Could you check a few things on this model? Use its own coordinates, in mm. Round coordinates to 2 decimals unless told otherwise and drop trailing zeros. Write each question's results on one line, items separated by ' | '. Start each with the question number.
(1) Imagine slicing it at A-A on z = 7.25. State how many separate pieces and enclosed holes the cut face has, then the cut area to 3 significant figures.
(2) Please list where these lines run through material, in increasing order: line 1 (Y direction, x = 162, z = 3); line 2 (X direction, y = 149.5, z = 6); line 3 (X direction, y = 140, z = 9.75). Write a range as [from, to].
(3) For P1, Ø1.8, axis at x = 130, y = 117.5, coming from the -Z side; P2, Ø3, axis at x = 179, z = 6, coming from the +Y side, each with a flat end and sliding along its axis, tell me the tip position at first contact or that it passes through.
```python
from build123d import *

# Parameters (mm, degrees)
F0_R     = 1.5
F1_DEPTH = 10


with BuildPart() as f1:
    # F0 (on Top) → F1 (new body)
    with BuildSketch(Plane.XY):
        Polygon((170, 158.5), (0, 158.5), (0, -91.5), (202, -91.5), (202, 100.5), (170, 100.5), align=None)
        with Locations((114, 101.5)):
            Circle(F0_R, mode=Mode.SUBTRACT)
        with Locations((114, 117.5)):
            Circle(F0_R, mode=Mode.SUBTRACT)
        with Locations((130, 101.5)):
            Circle(F0_R, mode=Mode.SUBTRACT)
        with Locations((146, 101.5)):
            Circle(F0_R, mode=Mode.SUBTRACT)
        with Locations((130, 117.5)):
            Circle(F0_R, mode=Mode.SUBTRACT)
        with Locations((146, 117.5)):
            Circle(F0_R, mode=Mode.SUBTRACT)
        with Locations((114, 133.5)):
            Circle(F0_R, mode=Mode.SUBTRACT)
        with Locations((114, 149.5)):
            Circle(F0_R, mode=Mode.SUBTRACT)
        with Locations((130, 133.5)):
            Circle(F0_R, mode=Mode.SUBTRACT)
        with Locations((146, 133.5)):
            Circle(F0_R, mode=Mode.SUBTRACT)
        with Locations((130, 149.5)):
            Circle(F0_R, mode=Mode.SUBTRACT)
        with Locations((146, 149.5)):
            Circle(F0_R, mode=Mode.SUBTRACT)
        with Locations((162, 101.5)):
            Circle(F0_R, mode=Mode.SUBTRACT)
        with Locations((162, 117.5)):
            Circle(F0_R, mode=Mode.SUBTRACT)
        with Locations((162, 133.5)):
            Circle(F0_R, mode=Mode.SUBTRACT)
        with Locations((162, 149.5)):
            Circle(F0_R, mode=Mode.SUBTRACT)
    extrude(amount=F1_DEPTH)


solid = f1.part
```
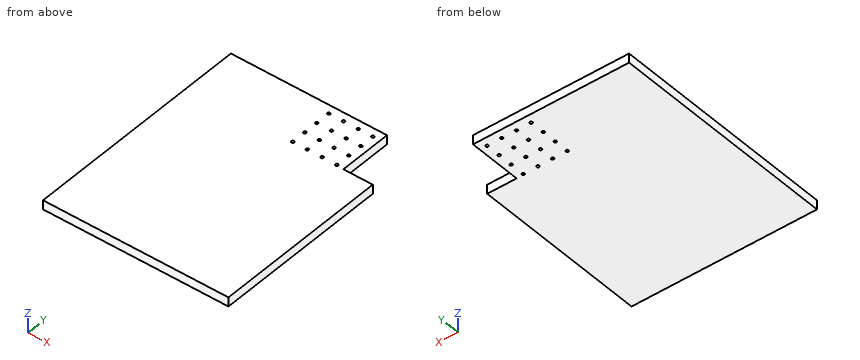
Response:
1) separate pieces: 1 | enclosed holes: 16 | area: 48,500 mm²
2) line 1: [-91.5, 100], [103, 116], [119, 132], [135, 148], [151, 158.5] | line 2: [0, 112.5], [115.5, 128.5], [131.5, 144.5], [147.5, 160.5], [163.5, 170] | line 3: [0, 170]
3) P1: through | P2: y = 100.5
